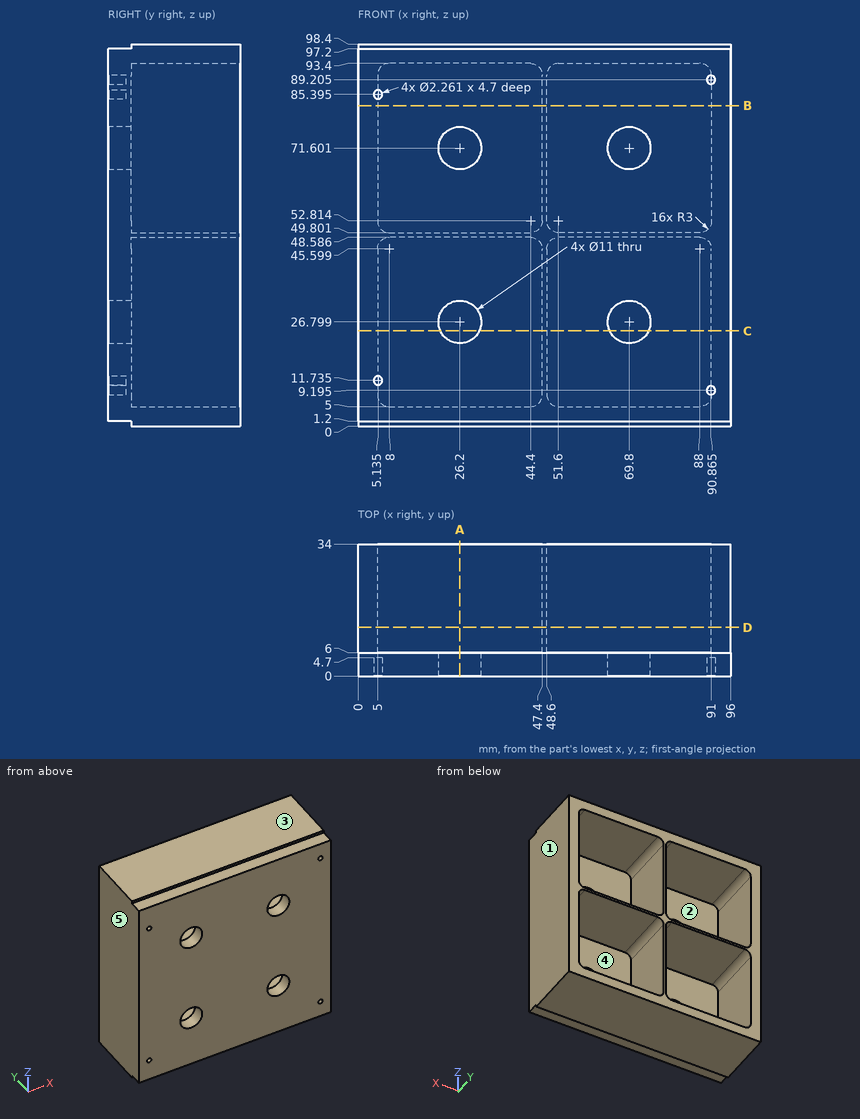
Geometry check sheet. Reference: drawing and pictorial views, mm from the part's lowest x, y, z. A direction names the side the tool comes from. Give positions to 0.01 mm unless a question says otherwise; leave off trailing zeros. Order: outer loops, then holes, each group sorted by start corner. A loop starts at its lowest first (then second) coordinate and runs counter-clockwise, first axis right, second up. Notation, with made-up numbers: M 73,44 L 101,44 A11 ccw 101,65 Z; hole C 48,-22.5 d2. An arc over 180 degrees is marked long. Answer as CSV lines item,"result". Start each with the question number.
Item 1: Cross-section at B-B on z = 82.5. Enter the section's corners in (x, y).
Item 2: Thickness scan on line 1 (Z direction, x = 28, y = 15); line 2 (X direction, y = 20, z = 74); line 3 (X direction, y = 32.5, z = 50.5) (1 decimal). Record the ranges inside material, lowest first. Write a range as [from, to].
Item 3: Mould release check, pull along Z, two halves, no side actions. Record for the marked faces 3, 4 and 5: +Z half, -Z half, draft (parallel to the pull), parting line (faces both ways), or undercut.
Item 4: Cross-section at D-D on y = 12.5. State how many separate pieces and enclosed holes the cut face has.
Item 5: Gauge pin test, flat ends, axial feed: P1, Ø3, axis at x = 12, z = 43.5, coming from the +Y side; P2, Ø1.1, axis at x = 91, z = 9, coming from the -Y side; P3, Ø1, axis at x = 47, z = 98, coming from the -Y side; P4, Ø6.5, axis at x = 69.8, z = 26.8, coming from the -Y side. Record the tip position at first contact, or that the pin passes through.
Item 6: Tool access check on the marked faces 1 and 2. Record the directions out of +Z, -Z, +X, -X, +Y, -Y that give a thin tool (end or side, any length) a straight path to the whole face; none if there is none.
Item 7: Cross-section at A-A on x = 26.2. Enter the section's corners in (y, z), plus the area to 3 significant figures.
Item 8: Cross-section at C-C on z = 24.5. Enter the section's corners in (x, y).
Established:
1,outline,"M 0,0 L 96,0 L 96,34 L 91,34 L 91,6 L 48.6,6 L 48.6,34 L 47.4,34 L 47.4,6 L 5,6 L 5,34 L 0,34 Z"
2,line 1,"z = [0, 5], [48.59, 49.81], [93.4, 98.4]"
2,line 2,"x = [0, 5], [47.4, 48.6], [91, 96]"
2,line 3,"x = [0, 6.1], [46.3, 49.7], [89.9, 96]"
3,face 3,"+Z half"
3,face 4,"undercut"
3,face 5,"draft"
4,separate pieces,"1"
4,enclosed holes,"4"
5,P1,"stops at y = 6"
5,P2,"stops at y = 4.7"
5,P3,"stops at y = 6"
5,P4,"passes through"
6,face 1,"+Z, -Z, +X, +Y, -Y"
6,face 2,"+Y"
7,outline,"M 0,1.2 L 6,1.2 L 6,0 L 34,0 L 34,5 L 6,5 L 6,21.3 L 0,21.3 Z; M 0,32.3 L 6,32.3 L 6,48.59 L 34,48.59 L 34,49.81 L 6,49.81 L 6,66.1 L 0,66.1 Z; M 0,77.1 L 6,77.1 L 6,93.4 L 34,93.4 L 34,98.4 L 6,98.4 L 6,97.2 L 0,97.2 Z"
7,area,"758 mm^2"
8,outline,"M 0,0 L 21.2,0 L 21.2,6 L 5,6 L 5,34 L 0,34 Z; M 31.2,0 L 64.8,0 L 64.8,6 L 48.6,6 L 48.6,34 L 47.4,34 L 47.4,6 L 31.2,6 Z; M 74.8,0 L 96,0 L 96,34 L 91,34 L 91,6 L 74.8,6 Z"
